Geometry: see drawing. Coordinates: mm, zero at the bounding-box minimum. A direction names the side the tool comes from. Give positions to 0.01 mm unless a question says otherwise; leave off trailing zeros. Write each loop counter-clockwise with the first axis right and the second up, starting at its lowest first coordinate (ties: lowest second). Pieces come first, ordered by that corner, then holes. Notation, with made-up numbers: (-30, 77) -> (0, 77) arc R30 cw to (0, 107) -> close; hole circle Ø1 at (56.25, 66). An arc over 180 degrees is marked (long way). Answer as a JSON object with one key per item and string values. Group by question number.
Item 1: Section query D-D on x = 13.5. Return the cut outline in (y, z), plus the area to 3 significant figures.
Item 2: First-contact query: pin 1 Ø8 at (x, y) = (9, 9) entering from -Z; pin 2 Ø1.5 at (y, z) = (5.5, 16) entering from +X. Flat tips, straight axial feed; report the tip coordinate or a pass-through.
Item 3: Pull-direction query (X, two-part tool) for the marked faces 1, 2 and 3; classes: pulls with the +X half, pulls with the -X half, needs draft (parallel to the pull), parting line crosses it, or undercut.
Item 4: Section query B-B on x = 9. Return the cut outline in (y, z).
Item 5: Section query C-C on z = 12.25. Return the cut outline in (x, y).
Item 6: Section query A-A on y = 9. Return the cut outline in (x, z), plus the area to 3 significant figures.
Item 7: Access query for the marked faces 4 and 5. Directions: +Z, -Z, +X, -X, +Y, -Y. A direction counts if a zero-diameter tool reaches every point of the face in a straight line with its end or side. Return the directions, or none.
Item 8: Ray query, probe 1 along Y at (x, z) = (9, 0.2); probe 2 along Z at (x, y) = (12.5, 6.5); probe 3 along Y at (x, z) = (6.25, 19.75). Return the intervals inside material, ascending. Write a range as from..to.
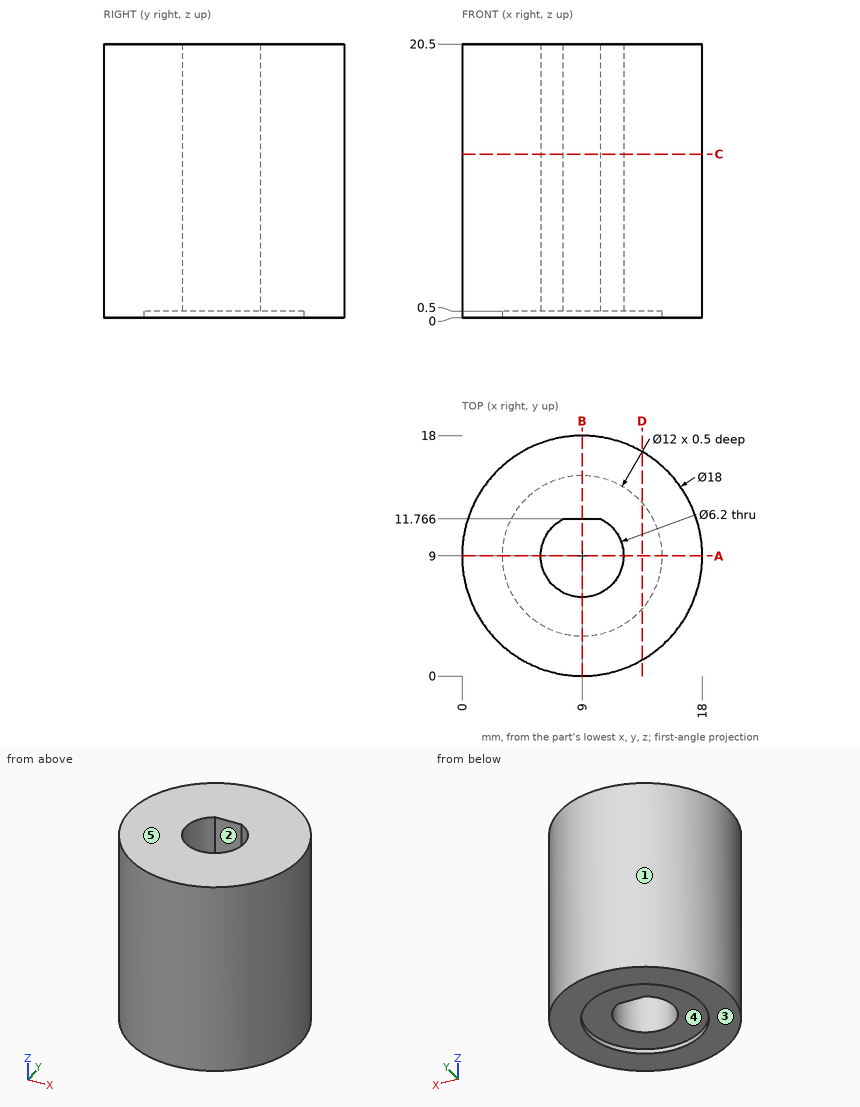
Worked answers:
{
 "1": {"outline": "(1.21, 0) -> (5.03, 0) -> (5.03, 0.5) -> (12.97, 0.5) -> (12.97, 0) -> (16.79, 0) -> (16.79, 20.5) -> (1.21, 20.5) -> close", "area": "316 mm^2"},
 "2": {"pin 1": "z = 0.5", "pin 2": "x = 17.57"},
 "3": {"face 1": "parting line crosses it", "face 2": "undercut", "face 3": "needs draft"},
 "4": {"outline": "(0, 0) -> (3, 0) -> (3, 0.5) -> (5.9, 0.5) -> (5.9, 20.5) -> (0, 20.5) -> close; (11.77, 0.5) -> (15, 0.5) -> (15, 0) -> (18, 0) -> (18, 20.5) -> (11.77, 20.5) -> close"},
 "5": {"outline": "circle Ø18 at (9, 9); hole (7.6, 11.77) arc R3.1 ccw (long way) to (10.4, 11.77) -> close"},
 "6": {"outline": "(0, 0) -> (3, 0) -> (3, 0.5) -> (5.9, 0.5) -> (5.9, 20.5) -> (0, 20.5) -> close; (12.1, 0.5) -> (15, 0.5) -> (15, 0) -> (18, 0) -> (18, 20.5) -> (12.1, 20.5) -> close", "area": "239 mm^2"},
 "7": {"face 4": "-Z", "face 5": "+Z, +X, -X, +Y, -Y"},
 "8": {"probe 1": "0..3, 15..18", "probe 2": "0.5..20.5", "probe 3": "0.43..7.57, 10.43..17.57"}
}
